```python
from build123d import *

# Parameters (mm, degrees)
SKETCH1_W           = 12.90052
SKETCH1_H           = 156.99994
SKETCH1_W_2         = 13
SKETCH1_R           = 2
BOSS_EXTRUDE1_DEPTH = 38.80104
CUT_EXTRUDE1_START  = 38.80104
SKETCH1_3_R         = 2
CUT_EXTRUDE1_DEPTH  = 6.35
SKETCH2_R           = 3.175
CUT_EXTRUDE2_DEPTH  = 12.7
CUT_EXTRUDE3_START  = -156.99994
SKETCH2_3_R         = 3.175
CUT_EXTRUDE3_DEPTH  = 12.7


with BuildPart() as part:
    # Sketch1 → Boss-Extrude1 (new body)
    with BuildSketch(Plane(origin=(0, 0, 0), x_dir=(1, 0, 0), z_dir=(0, 1, 0))):
        with Locations((-6.45026, 78.49997)):
            Rectangle(SKETCH1_W, SKETCH1_H)
        with Locations((6.5, 78.49997)):
            Rectangle(SKETCH1_W_2, SKETCH1_H)
        with Locations((6.5, 20)):
            Circle(SKETCH1_R, mode=Mode.SUBTRACT)
        with Locations((6.5, 79.944)):
            Circle(SKETCH1_R, mode=Mode.SUBTRACT)
        with Locations((6.5, 139.888)):
            Circle(SKETCH1_R, mode=Mode.SUBTRACT)
        with Locations((19.45026, 78.49997)):
            Rectangle(SKETCH1_W, SKETCH1_H)
        with Locations((6.5, 20)):
            Circle(SKETCH1_R)
        with Locations((6.5, 139.888)):
            Circle(SKETCH1_R)
        with Locations((6.5, 79.944)):
            Circle(SKETCH1_R)
    extrude(amount=BOSS_EXTRUDE1_DEPTH)

    # Sketch1<3> → Cut-Extrude1 (cut)
    with BuildSketch(Plane(origin=(0, 0, 0), x_dir=(1, 0, 0), z_dir=(0, 1, 0)).offset(CUT_EXTRUDE1_START)):
        with Locations((6.5, 20)):
            Circle(SKETCH1_3_R)
        with Locations((6.5, 79.944)):
            Circle(SKETCH1_3_R)
        with Locations((6.5, 139.888)):
            Circle(SKETCH1_3_R)
    extrude(amount=-CUT_EXTRUDE1_DEPTH, mode=Mode.SUBTRACT)

    # Sketch2 → Cut-Extrude2 (cut)
    with BuildSketch(Plane.XY):
        with Locations((-6.55052, 32.45104)):
            Circle(SKETCH2_R)
        with Locations((19.55052, 32.45104)):
            Circle(SKETCH2_R)
        with Locations((19.55052, 6.35)):
            Circle(SKETCH2_R)
        with Locations((-6.55052, 6.35)):
            Circle(SKETCH2_R)
    extrude(amount=-CUT_EXTRUDE2_DEPTH, mode=Mode.SUBTRACT)

    # Sketch2<3> → Cut-Extrude3 (cut)
    with BuildSketch(Plane.XY.offset(CUT_EXTRUDE3_START)):
        with Locations((-6.55052, 32.45104)):
            Circle(SKETCH2_3_R)
        with Locations((19.55052, 32.45104)):
            Circle(SKETCH2_3_R)
        with Locations((19.55052, 6.35)):
            Circle(SKETCH2_3_R)
        with Locations((-6.55052, 6.35)):
            Circle(SKETCH2_3_R)
    extrude(amount=CUT_EXTRUDE3_DEPTH, mode=Mode.SUBTRACT)


solid = part.part
```
The model under review builds one solid part; all positions refer to its coordinate system, in mm. A direction names the side the tool comes from. Round coordinates to 2 decimals unless told otherwise and drop trailing zeros. Loops run counter-clockwise (first coordinate to the right, second up) from the corner with the lowest first, then second, coordinate; pieces in that order, holes last. Notation, with made-up numbers: M 24,18.25 L 55,18.25 A17 cw 55,39.25 Z; hole C 15.5,54 d5. An arc over 180 degrees is marked long. Answer as a JSON object with one key per item and string values.
(1) Take a section at A-A on z = -20. Give the boundary of the cut face in (x, y).
Resolved:
{"outline": "M -12.9,0 L 25.9,0 L 25.9,38.8 L 8.5,38.8 L 8.5,32.45 L 4.5,32.45 L 4.5,38.8 L -12.9,38.8 Z"}
(2) Take a section at B-B on y = 6.35. Give the boundary of the cut face in (x, z).
Resolved:
{"outline": "M -12.9,-157 L -9.73,-157 L -9.73,-144.3 L -3.38,-144.3 L -3.38,-157 L 16.38,-157 L 16.38,-144.3 L 22.73,-144.3 L 22.73,-157 L 25.9,-157 L 25.9,0 L 22.73,0 L 22.73,-12.7 L 16.38,-12.7 L 16.38,0 L -3.38,0 L -3.38,-12.7 L -9.73,-12.7 L -9.73,0 L -12.9,0 Z"}
(3) Tool access review of faces 5 (the cylindrical face through (16.38, 32.59, -150.74)), 6 (the cylindrical face through (-4.8, 35.1, -6.3)), 7 (the cylindrical face through (6.07, 35.67, -77.99)): name each direction out of +Z, -Z, +X, -X, +Y, -Y from which nothing blocks a thin tool from reaching the whole face with its end or side.
Resolved:
{"face 5": "-Z", "face 6": "+Z", "face 7": "+Y"}
(4) Draft analysis for pull direction Z (two halves, no side actions). For faces 1 (the flat face through (6, 32.451, -20)), 2 (the cylindrical face through (-6.96, 9.5, -150.74)), 3 (the flat face through (-7, 6, -12.7)), 4 (the flat face through (20, 6, -144.3)), state which applies: released by +Z, released by -Z, zero draft, split by the parting line, or undercut.
Resolved:
{"face 1": "undercut", "face 2": "zero draft", "face 3": "released by +Z", "face 4": "released by -Z"}
(5) To check wall thickness, follow line 1 along X through (y, z) = (6, -148); line 2 along X through (y, z) = (34, -20); line 3 along Z through (x, y) = (6, 37). State the ranges of each line that lie inside material, in increasing order.
Resolved:
{"line 1": "-12.9 to -9.71, -3.39 to 16.39, 22.71 to 25.9", "line 2": "-12.9 to 4.5, 8.5 to 25.9", "line 3": "-157 to -141.82, -137.95 to -81.88, -78.01 to -21.94, -18.06 to 0"}
(6) Take a section at C-C on x = -6. Give the boundary of the cut face in (y, z).
Resolved:
{"outline": "M 0,-157 L 3.22,-157 L 3.22,-144.3 L 9.48,-144.3 L 9.48,-157 L 29.32,-157 L 29.32,-144.3 L 35.58,-144.3 L 35.58,-157 L 38.8,-157 L 38.8,0 L 35.58,0 L 35.58,-12.7 L 29.32,-12.7 L 29.32,0 L 9.48,0 L 9.48,-12.7 L 3.22,-12.7 L 3.22,0 L 0,0 Z"}
(7) Clearance check with flat-ended pins moving along their axes: P1, Ø5, axis at x = -6.55, y = 6.35, coming from the -Z side; P2, Ø1.9, axis at x = -5, y = 34, coming from the +Z side. State where each tip first meets the part, or that it passes through.
Resolved:
{"P1": "z = -144.3", "P2": "z = -12.7"}
